from build123d import *

# Parameters (mm, degrees)
F0_W     = 4.6
F0_H     = 4.8
F0_W_2   = 35.4
F1_DEPTH = 2.3
F0_W_3   = 45.2
F0_H_2   = 59.6
F0_W_4   = 0.2
F2_DEPTH = 3.5
F3_DEPTH = 7.7


with BuildPart() as f1:
    # F0 (on Top) → F1 (new body, symmetric)
    with BuildSketch(Plane.XY):
        Polygon((19.5689408898, 51.453421098), (-27.7310591102, 51.453421098), (-27.7310591102, -17.746578902), (19.5689408898, -17.746578902), (19.5689408898, -12.946578902), (-25.6310591102, -12.946578902), (-25.6310591102, 46.653421098), (19.5689408898, 46.653421098), align=None)
        with Locations((21.8689408898, 49.053421098)):
            Rectangle(F0_W, F0_H)
        with Locations((41.8689408898, 49.053421098)):
            Rectangle(F0_W_2, F0_H)
        with Locations((61.8689408898, 49.053421098)):
            Rectangle(F0_W, F0_H)
        with Locations((21.8689408898, -15.346578902)):
            Rectangle(F0_W, F0_H)
        with Locations((41.8689408898, -15.346578902)):
            Rectangle(F0_W_2, F0_H)
        with Locations((61.8689408898, -15.346578902)):
            Rectangle(F0_W, F0_H)
    extrude(amount=F1_DEPTH, both=True)

    # F0 (on Top) → F2 (join, symmetric)
    with BuildSketch(Plane.XY):
        with Locations((-3.0310591102, 16.853421098)):
            Rectangle(F0_W_3, F0_H_2)
        with Locations((21.8689408898, 16.853421098)):
            Rectangle(F0_W, F0_H_2)
        with Locations((41.8689408898, 16.853421098)):
            Rectangle(F0_W_2, F0_H_2)
        with Locations((61.8689408898, 16.853421098)):
            Rectangle(F0_W, F0_H_2)
        with Locations((64.2689408898, 16.853421098)):
            Rectangle(F0_W_4, F0_H_2)
    extrude(amount=F2_DEPTH, both=True)

    # F0 (on Top) → F3 (join)
    with BuildSketch(Plane.XY):
        with Locations((21.8689408898, 16.853421098)):
            Rectangle(F0_W, F0_H_2)
        with Locations((21.8689408898, 49.053421098)):
            Rectangle(F0_W, F0_H)
        with Locations((21.8689408898, -15.346578902)):
            Rectangle(F0_W, F0_H)
        with Locations((61.8689408898, -15.346578902)):
            Rectangle(F0_W, F0_H)
        with Locations((61.8689408898, 16.853421098)):
            Rectangle(F0_W, F0_H_2)
        with Locations((61.8689408898, 49.053421098)):
            Rectangle(F0_W, F0_H)
    extrude(amount=-F3_DEPTH)


solid = f1.part
Work out the finished part from the listing and answer in its coordinate system (mm). A direction names the side the tool comes from. Round coordinates to 2 decimals unless told otherwise and drop trailing zeros. Write each loop counter-clockwise with the first axis right and the second up, starting at its lowest first coordinate (ties: lowest second). Pieces come first, ordered by that corner, then holes.
1) The mould has two halves that part along X. Classify faces 6 (the flat face through (19, 51.453, 0)), 7 (the flat face through (42, 49, -2.3)), 8 (the flat face through (64.369, 16, 0)): pulls with the +X half, pulls with the -X half, needs draft (parallel to the pull), parting line crosses it, or undercut.
2) Straight lines are drawn through the part: line 1 (X direction, y = 35, z = -6.75); line 2 (Z direction, x = -17.5, y = 28.5); line 3 (Z direction, x = 59.5, y = -14.5). For each, find the intervals that lie inside material, in ascending order.
3) Given pin 1 Ø1.3 at (x, z) = (-3.5, -3) entering from +Y; pin 2 Ø1 at (x, y) = (25.5, 27.5) entering from -Z; pin 3 Ø1.3 at (x, z) = (44.5, -3) entering from -Y, each flat-ended and moving along its own axis, determine where each tip first touches the part or whether it passes through.
4) A cutting plane is placed at B-B (x = -18.5). Give the vertices of the cut face in (y, z), plus the area to 3 significant figures.
5) A cutting plane is placed at C-C (y = 18.5). Give the vertices of the cut face in (x, z), plus the area to 3 significant figures.
6) A tool of negligible diameter and unlimited length cuts with its end or side. For faces 1 (the flat face through (22, 17, -7.7)), 2 (the flat face through (-3, 17, -3.5)), 3 (the flat face through (18, -17.747, 1)), 4 (the flat face through (42, -15, -2.3)), 5 (the flat face through (42, 17, -3.5)), from which of +Z, -Z, +X, -X, +Y, -Y can it reach the whole face along a straight path? Write none if from no direction.
7) A cutting plane is placed at A-A (z = -5.5). Give the vertices of the cut face in (x, y).
Completed:
1. face 6: needs draft
1. face 7: undercut
1. face 8: pulls with the +X half
2. line 1: x = 19.57 to 24.17, 59.57 to 64.17
2. line 2: z = -3.5 to 3.5
2. line 3: z = -2.3 to 2.3
3. pin 1: stops at y = 46.65
3. pin 2: stops at z = -3.5
3. pin 3: stops at y = -12.95
4. outline: (-17.75, -2.3) - (-12.95, -2.3) - (-12.95, -3.5) - (46.65, -3.5) - (46.65, -2.3) - (51.45, -2.3) - (51.45, 2.3) - (46.65, 2.3) - (46.65, 3.5) - (-12.95, 3.5) - (-12.95, 2.3) - (-17.75, 2.3) - close
4. area: 461 mm2
5. outline: (-27.73, -2.3) - (-25.63, -2.3) - (-25.63, -3.5) - (19.57, -3.5) - (19.57, -7.7) - (24.17, -7.7) - (24.17, -3.5) - (59.57, -3.5) - (59.57, -7.7) - (64.17, -7.7) - (64.17, -3.5) - (64.37, -3.5) - (64.37, 3.5) - (-25.63, 3.5) - (-25.63, 2.3) - (-27.73, 2.3) - close
5. area: 678 mm2
6. face 1: -Z, +X, -X, +Y, -Y
6. face 2: -Z, -X, +Y, -Y
6. face 3: +Z, -Z, +X, -X, -Y
6. face 4: -Z, -Y
6. face 5: -Z, +Y, -Y
7. outline: (19.57, -17.75) - (24.17, -17.75) - (24.17, 51.45) - (19.57, 51.45) - close; (59.57, -17.75) - (64.17, -17.75) - (64.17, 51.45) - (59.57, 51.45) - close
